Check sheet for the modelled part. Datum: model origin and axes. Units: mm. Round coordinates to 2 decimals unless told otherwise and drop trailing zeros. Write each loop counter-clockwise with the first axis right and the second up, starting at its lowest first coordinate (ties: lowest second). Pieces come first, ordered by that corner, then holes. Notation, with made-up numbers: M 13.25,7 L 42.25,7 A35 ccw 42.25,41 Z; hole C 29.25,-20.5 d6. An arc over 180 degrees is marked long. One line per item, written item: value.
from build123d import *

# Parameters (mm, degrees)
SKETCH_1_W          = 14.73
SKETCH_1_H          = 15.24
EXTRUDE_1_DEPTH     = 1.6
SKETCH_2_R          = 0.55
CUT_EXTRUDE_1_DEPTH = 11.717631501
CUT_EXTRUDE_2_DEPTH = 0.0001


with BuildPart() as part:
    # Эскиз1 → Бобышка-Вытянуть1 (new body)
    with BuildSketch(Plane(origin=(0, 0, 0), x_dir=(1, 0, 0), z_dir=(0, 1, 0))):
        Rectangle(SKETCH_1_W, SKETCH_1_H)
    extrude(amount=EXTRUDE_1_DEPTH)

    # Эскиз2 → Вырез-Вытянуть1 (cut, through all)
    with BuildSketch(Plane(origin=(0, 1.6, 0), x_dir=(1, 0, 0), z_dir=(0, 1, 0))):
        with Locations(Location((-4.825, 6, 0), (0, 0, 270))):
            Circle(SKETCH_2_R)
        with Locations(Location((-2.285, 6, 0), (0, 0, 270))):
            Circle(SKETCH_2_R)
        with Locations(Location((-4.8, -6.07, 0), (0, 0, 270))):
            Circle(SKETCH_2_R)
        with Locations(Location((-2.260000197, -6.071, 0), (0, 0, 270))):
            Circle(SKETCH_2_R)
    extrude(amount=-CUT_EXTRUDE_1_DEPTH, mode=Mode.SUBTRACT)

    # Эскиз3 → Вырез-Вытянуть2 (cut)
    with BuildSketch(Plane(origin=(0, 1.6, 0), x_dir=(1, 0, 0), z_dir=(0, 1, 0))):
        with BuildLine():
            Line((-6.729, 3.627), (-5.809, 3.627))
            ThreePointArc((-5.809, 3.627), (-5.509, 3.327), (-5.809, 3.027))
            Line((-5.809, 3.027), (-6.729, 3.027))
            ThreePointArc((-6.729, 3.027), (-7.029, 3.327), (-6.729, 3.627))
        make_face()
        with BuildLine():
            Line((-6.729, 2.357), (-5.809, 2.357))
            ThreePointArc((-5.809, 2.357), (-5.509, 2.057), (-5.809, 1.757))
            Line((-5.809, 1.757), (-6.729, 1.757))
            ThreePointArc((-6.729, 1.757), (-7.029, 2.057), (-6.729, 2.357))
        make_face()
        with BuildLine():
            Line((-6.729, 1.087), (-5.809, 1.087))
            ThreePointArc((-5.809, 1.087), (-5.509, 0.787), (-5.809, 0.487))
            Line((-5.809, 0.487), (-6.729, 0.487))
            ThreePointArc((-6.729, 0.487), (-7.029, 0.787), (-6.729, 1.087))
        make_face()
        with BuildLine():
            Line((-6.729, -0.183), (-5.809, -0.183))
            ThreePointArc((-5.809, -0.183), (-5.509, -0.483), (-5.809, -0.783))
            Line((-5.809, -0.783), (-6.729, -0.783))
            ThreePointArc((-6.729, -0.783), (-7.029, -0.483), (-6.729, -0.183))
        make_face()
        with BuildLine():
            Line((-1.249, 2.357), (-0.329, 2.357))
            ThreePointArc((-0.329, 2.357), (-0.029, 2.057), (-0.329, 1.757))
            Line((-0.329, 1.757), (-1.249, 1.757))
            ThreePointArc((-1.249, 1.757), (-1.549, 2.057), (-1.249, 2.357))
        make_face()
        with BuildLine():
            Line((-1.249, 1.087), (-0.329, 1.087))
            ThreePointArc((-0.329, 1.087), (-0.029, 0.787), (-0.329, 0.487))
            Line((-0.329, 0.487), (-1.249, 0.487))
            ThreePointArc((-1.249, 0.487), (-1.549, 0.787), (-1.249, 1.087))
        make_face()
        with BuildLine():
            Line((-1.249, -0.183), (-0.329, -0.183))
            ThreePointArc((-0.329, -0.183), (-0.029, -0.483), (-0.329, -0.783))
            Line((-0.329, -0.783), (-1.249, -0.783))
            ThreePointArc((-1.249, -0.783), (-1.549, -0.483), (-1.249, -0.183))
        make_face()
        with BuildLine():
            Line((-1.249, 3.627), (-0.329, 3.627))
            ThreePointArc((-0.329, 3.627), (-0.029, 3.327), (-0.329, 3.027))
            Line((-0.329, 3.027), (-1.249, 3.027))
            ThreePointArc((-1.249, 3.027), (-1.549, 3.327), (-1.249, 3.627))
        make_face()
    extrude(amount=-CUT_EXTRUDE_2_DEPTH, mode=Mode.SUBTRACT)


solid = part.part
Q1. Sectioned sample at A-A on z = 6.07. Enter the section's corners in (x, y) (3 decimals).
Completed:
outline: M -7.365,0 L -5.35,0 L -5.35,1.6 L -7.365,1.6 Z; M -4.25,0 L -2.81,0 L -2.81,1.6 L -4.25,1.6 Z; M -1.71,0 L 7.365,0 L 7.365,1.6 L -1.71,1.6 Z
Q2. Scan lines: line 1 (Z direction, x = -4.75, y = 1.2); line 2 (X direction, y = 0.65, z = 6) (3 decimals); line 3 (X direction, y = 1.05, z = -6) (3 decimals). Record each from-to range of solid material in increasing order. Write a range as [from, to].
Completed:
line 1: [-7.62, -6.54], [-5.46, 5.52], [6.62, 7.62]
line 2: [-7.365, -5.346], [-4.254, -2.805], [-1.715, 7.365]
line 3: [-7.365, -5.375], [-4.275, -2.835], [-1.735, 7.365]
Q3. Sectioned sample at B-B on y = 1.4. Enter the section's corners in (x, z) (3 decimals), and give its area (3 significant figures).
Completed:
outline: M -7.365,-7.62 L 7.365,-7.62 L 7.365,7.62 L -7.365,7.62 Z; hole C -4.825,-6 d1.1; hole C -4.8,6.07 d1.1; hole C -2.285,-6 d1.1; hole C -2.26,6.071 d1.1
area: 221 mm^2
Q4. Draft check along X on faces 1 (the cylindrical face through (-5.01, 0.81, 6.58)), 2 (the flat face through (7.365, 1, 0)), 3 (the cylindrical face through (-2.496, 0.811, -5.492)), 4 (the flat face through (0, 0, 0)). Enter one of: pulls with the +X half, pulls with the -X half, needs draft (parallel to the pull), parting line crosses it, or undercut.
Completed:
face 1: undercut
face 2: pulls with the +X half
face 3: undercut
face 4: needs draft
